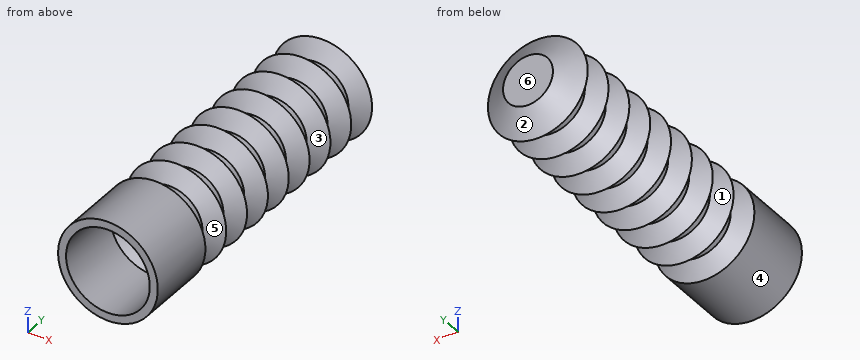
from build123d import *


with BuildPart() as part:
    # Sketch1 → Revolve6 (revolve)
    with BuildSketch(Plane.XY, mode=Mode.PRIVATE) as revolve6_sk:
        Polygon((-0.431630681, 32.7), (-2.131630681, 31.68), (-2.131630681, 30.54), (-0.431630681, 29.52), (-2.131630681, 28.5), (-2.131630681, 27.36), (-0.431630681, 26.34), (-2.131630681, 25.32), (-2.131630681, 24.18), (-0.431630681, 23.16), (-2.131630681, 22.14), (-2.131630681, 21), (-0.431630681, 19.98), (-2.131630681, 18.96), (-2.131630681, 17.82), (-0.431630681, 16.8), (-2.131630681, 15.78), (-2.131630681, 14.64), (-0.431630681, 13.62), (-2.131630681, 12.6), (-2.131630681, 11.46), (-0.431630681, 10.44), (-2.131630681, 9.42), (-2.131630681, 8.28), (-0.431630681, 7.26), (-0.431630681, 0), (-1.231630681, 0), (-1.231630681, 6.795995819), (-1.995791511, 7.26), (-3.138866015, 7.96), (-3.138866015, 9.754155298), (-1.995791511, 10.44), (-3.138866015, 11.14), (-3.138866015, 12.934155298), (-1.995791511, 13.62), (-3.138866015, 14.32), (-3.138866015, 16.114155298), (-1.995791511, 16.8), (-3.138866015, 17.5), (-3.138866015, 19.294155298), (-1.995791511, 19.98), (-3.138866015, 20.68), (-3.138866015, 22.474155298), (-1.995791511, 23.16), (-3.138866015, 23.86), (-3.138866015, 25.654155298), (-1.995791511, 26.34), (-3.138866015, 27.04), (-3.138866015, 28.834155298), (-1.995791511, 29.52), (-3.138866015, 30.22), (-3.138866015, 32.014155298), (-1.995791511, 32.7), (-3.138866015, 33.4), (-5.431630681, 33.4), (-5.431630681, 34.2), (-2.931630681, 34.2), align=None)
    revolve(revolve6_sk.sketch.rotate(Axis((-5.431630681, 34.2, 0), (0, -1, 0)), 180), axis=Axis((-5.431630681, 34.2, 0), (0, -1, 0)))


solid = part.part
The model under review builds one solid part; all positions refer to its coordinate system, in mm. Face numbers are marked on the shaded views. A direction names the side the tool comes from. Round coordinates to 2 decimals unless told otherwise and drop trailing zeros. Answer as a JSON object with one key per item and string values.
Item 1: Tool access review of the marked faces 5 and 6: name each direction out of +Z, -Z, +X, -X, +Y, -Y from which nothing blocks a thin tool from reaching the whole face with its end or side.
Check sheet entries:
{"face 5": "none", "face 6": "+Z, -Z, +X, -X, +Y"}
Item 2: Clearance check with flat-ended pins moving along their axes: P1, Ø4, axis at x = -5.43, z = 0, coming from the -Y side; P2, Ø5.5, axis at x = -5.43, z = 0, coming from the -Y side; P3, Ø1.5, axis at x = -5, y = 13, coming from the +Z side; P4, Ø6, axis at x = -5.43, z = 0, coming from the -Y side. State where each tip first meets the part, or that it passes through.
Check sheet entries:
{"P1": "y = 33.4", "P2": "y = 7.68", "P3": "z = 5", "P4": "y = 7.53"}
Item 3: For line 1 along Y through (x, z) = (-5.5, -2.25); line 2 along Z through (x, y) = (-7.5, 24); line 3 along Z through (x, y) = (-5.25, 19.5), list the stretches that pass through material, from the lowest coordinate up.
Check sheet entries:
{"line 1": "33.4 to 34.2", "line 2": "-2.95 to -0.99, 0.99 to 2.95", "line 3": "-4.2 to -2.63, 2.63 to 4.2"}
Item 4: The part is to be moulded in two halves that separate along Y. For the marked faces 1, 2, 3 and 4, say which applies: +Y half, -Y half, draft (parallel to the pull), parting line (faces both ways), or undercut.
Check sheet entries:
{"face 1": "undercut", "face 2": "+Y half", "face 3": "undercut", "face 4": "draft"}
